Read the model definition and answer for the solid it produces. Units are mm, in the model's axes. A direction names the side the tool comes from. Round coordinates to 2 decimals unless told otherwise and drop trailing zeros. Loops run counter-clockwise (first coordinate to the right, second up) from the corner with the lowest first, then second, coordinate; pieces in that order, holes last. Notation, with made-up numbers: (8, 50.5) -> (56, 50.5) arc R21 ccw to (56, 88.5) -> close; hole circle Ø2 at (-5, -15.5). An arc over 180 degrees is marked (long way). Put each result on its own line as item: value.
from build123d import *

# Parameters (mm, degrees)
SKETCH1_W                                            = 114.3
SKETCH1_H                                            = 63.5
BOSS_EXTRUDE1_DEPTH                                  = 15.24
F_5_8_0_625_DIAMETER_HOLE1_D                         = 15.875
F_10_24_TAPPED_HOLE3_D                               = 3.7973
CBORE_FOR_3_8_BINDING_HEAD_MACHINE_SCREW_D           = 9.5758
CBORE_FOR_3_8_BINDING_HEAD_MACHINE_SCREW_CBORE_D     = 19.05
CBORE_FOR_3_8_BINDING_HEAD_MACHINE_SCREW_CBORE_DEPTH = 7.62
F_10_24_TAPPED_HOLE1_D                               = 3.7973
F_10_24_TAPPED_HOLE1_DEPTH                           = 10.035175986
F_10_24_TAPPED_HOLE1_TIP                             = 1.140824014
F_10_24_TAPPED_HOLE2_D                               = 3.7973
F_10_24_TAPPED_HOLE2_DEPTH                           = 10.035175986
F_10_24_TAPPED_HOLE2_TIP                             = 1.140824014
FILLET1_R                                            = 1.27


with BuildPart() as part:
    # Sketch1 → Boss-Extrude1 (new body)
    with BuildSketch(Plane(origin=(0, 0, 0), x_dir=(1, 0, 0), z_dir=(0, 1, 0))):
        with Locations((-6.35, 0)):
            Rectangle(SKETCH1_W, SKETCH1_H)
    extrude(amount=BOSS_EXTRUDE1_DEPTH)

    # 5/8 (0.625) Diameter Hole1 (through all)
    with Locations(Plane(origin=(0, 15.24, 0), x_dir=(1, 0, 0), z_dir=(0, 1, 0))):
        with Locations((-31.75, 0)):
            Hole(F_5_8_0_625_DIAMETER_HOLE1_D / 2)

    # #10-24 Tapped Hole3 (through all)
    with Locations(Plane(origin=(0, 15.24, 0), x_dir=(1, 0, 0), z_dir=(0, 1, 0))):
        with Locations((-24.60625, -12.373337957), (-24.60625, 12.373337957)):
            Hole(F_10_24_TAPPED_HOLE3_D / 2)

    # CBORE for 3/8 Binding Head Machine Screw1 (through all)
    with Locations(Plane(origin=(0, 0, 0), x_dir=(-1, 0, 0), z_dir=(0, -1, 0))):
        with Locations((-31.75, 0)):
            CounterBoreHole(CBORE_FOR_3_8_BINDING_HEAD_MACHINE_SCREW_D / 2, CBORE_FOR_3_8_BINDING_HEAD_MACHINE_SCREW_CBORE_D / 2, CBORE_FOR_3_8_BINDING_HEAD_MACHINE_SCREW_CBORE_DEPTH)

    # #10-24 Tapped Hole1
    with Locations(Plane(origin=(0, 0, -31.75), x_dir=(-1, 0, 0), z_dir=(0, 0, -1))):
        with Locations((49.657, 7.62), (1.397, 7.62)):
            Hole(F_10_24_TAPPED_HOLE1_D / 2, depth=F_10_24_TAPPED_HOLE1_DEPTH)
            with Locations((0, 0, -(F_10_24_TAPPED_HOLE1_DEPTH + F_10_24_TAPPED_HOLE1_TIP / 2))):  # 118° drill point
                Cone(0, F_10_24_TAPPED_HOLE1_D / 2, F_10_24_TAPPED_HOLE1_TIP, mode=Mode.SUBTRACT)

    # #10-24 Tapped Hole2
    with Locations(Plane.XY.offset(31.75)):
        with Locations((-49.657, 7.62), (-1.397, 7.62)):
            Hole(F_10_24_TAPPED_HOLE2_D / 2, depth=F_10_24_TAPPED_HOLE2_DEPTH)
            with Locations((0, 0, -(F_10_24_TAPPED_HOLE2_DEPTH + F_10_24_TAPPED_HOLE2_TIP / 2))):  # 118° drill point
                Cone(0, F_10_24_TAPPED_HOLE2_D / 2, F_10_24_TAPPED_HOLE2_TIP, mode=Mode.SUBTRACT)

    # Fillet1
    fillet1_edges = [part.edges().sort_by_distance(p)[0] for p in [
        (50.8, 7.62, -31.75),
        (-63.5, 7.62, -31.75),
        (-63.5, 7.62, 31.75),
        (50.8, 7.62, 31.75),
    ]]
    fillet(fillet1_edges, radius=FILLET1_R)


solid = part.part
Item 1: Flat-ended cylindrical pins translate along their axes: pin 1 Ø2.5 at (x, z) = (-24.61, -12.37) entering from -Y; pin 2 Ø5.5 at (x, z) = (28, -4) entering from -Y; pin 3 Ø3 at (x, y) = (-1.397, 7.62) entering from +Z; pin 4 Ø3.5 at (x, y) = (-49.657, 7.62) entering from -Z. Find the tip coordinate at first contact, or state that the pin passes through.
Derived:
pin 1: passes through
pin 2: stops at y = 7.62
pin 3: stops at z = 21.48
pin 4: stops at z = -21.63
Item 2: The part is cut by section A-A (z = 0). Determine the outline of the cut face in (x, y) (1 decimal).
Derived:
outline: (-63.5, 0) -> (-39.7, 0) -> (-39.7, 15.2) -> (-63.5, 15.2) -> close; (-23.8, 0) -> (22.2, 0) -> (22.2, 7.6) -> (27, 7.6) -> (27, 15.2) -> (-23.8, 15.2) -> close; (36.5, 7.6) -> (41.3, 7.6) -> (41.3, 0) -> (50.8, 0) -> (50.8, 15.2) -> (36.5, 15.2) -> close
Item 3: Which of the six approach directions +Z, -Z, +X, -X, +Y, -Y give full straight-line access (tool end or side, diameter ignored) to faces 1 (the cylindrical face through (-49.904, 9.502, -26.662)), 2 (the cylindrical face through (-50.68, 9.22, 26.66)), 3 (the flat face through (-7, 15.24, 0)), 4 (the cylindrical face through (41.266, 3.757, -0.419))?
Derived:
face 1: -Z
face 2: +Z
face 3: +Z, -Z, +X, -X, +Y
face 4: -Y
Item 4: For a pull along Z with two mould halves and no side action, classify faces 5 (the flat face through (34, 7.62, -4.4)), 6 (the conical face through (-49.97, 7.72, -20.77)), 7 (the flat face through (-63.5, 8, 0)), 8 (the flat face through (-7, 8, 31.75)) as pulls with the +Z half, pulls with the -Z half, needs draft (parallel to the pull), parting line crosses it, or undercut.
Derived:
face 5: undercut
face 6: pulls with the -Z half
face 7: needs draft
face 8: pulls with the +Z half
Item 5: The part is cut by section B-B (x = 31.75). Determine the outline of the cut face in (y, z) (3 decimals).
Derived:
outline: (0, -31.75) -> (15.24, -31.75) -> (15.24, -4.788) -> (7.62, -4.788) -> (7.62, -9.525) -> (0, -9.525) -> close; (0, 9.525) -> (7.62, 9.525) -> (7.62, 4.788) -> (15.24, 4.788) -> (15.24, 31.75) -> (0, 31.75) -> close
Item 6: The part is cut by section C-C (y = 4.25). State how many separate pieces and enclosed holes the cut face has, then the cut area to 3 significant figures.
Derived:
separate pieces: 1
enclosed holes: 4
area: 6,750 mm^2
Item 7: The part is cut by section D-D (x = -31.75). Determine the outline of the cut face in (y, z), then the cut area to 3 significant figures.
Derived:
outline: (0, -31.75) -> (15.24, -31.75) -> (15.24, -7.94) -> (0, -7.94) -> close; (0, 7.94) -> (15.24, 7.94) -> (15.24, 31.75) -> (0, 31.75) -> close
area: 726 mm^2
Item 8: Find the intervals of material crossed by line 1 along X through (y, z) = (7.62, 27); line 2 along Z through (x, y) = (-31.75, 10.5); line 3 along X through (y, z) = (6, 28), in increasing order.
Derived:
line 1: x = -63.5 to -51.56, -47.76 to -3.3, 0.5 to 50.8
line 2: z = -31.75 to -7.94, 7.94 to 31.75
line 3: x = -63.5 to -50.65, -48.67 to -2.39, -0.41 to 50.8
